Design review of the part built by this model. Coordinates are the model's own, in mm. Face numbers are marked on the shaded views. A direction names the side the tool comes from. Coordinates: 2 decimals unless noted, no trailing zeros. Write each loop counter-clockwise with the first axis right and the second up, starting at its lowest first coordinate (ties: lowest second). Pieces come first, ordered by that corner, then holes.
Q1. To check wall thickness, follow probe 1 along X at (y, z) = (5.25, -7.5); probe 2 along Y at (x, z) = (0, -1); probe 3 along X at (y, z) = (19.5, 9). State the ranges of each line that lie inside material, in increasing order.
Q2. Add section B-B, the plane z = 7.5. Give the boundary of the cut face in (x, y), plus the area to 3 significant figures.
Q3. Add section C-C, the plane y = 5.5. Give the number of separate pieces and of enclosed holes in the cut face, plus the area to 3 significant figures.
Q4. Machinability: for the marked faces 1 and 2, which of the approach directions +Z, -Z, +X, -X, +Y, -Y give a long, thin tool a straight path to every point of the face, cutting with its end or side? Answer none if there is none.
Q5. Add section A-A, the plane x = 0. Give the boundary of the cut face in (y, z).
Q6. Clearance check with flat-ended pins moving along their axes: pin 1 Ø0.6 at (x, z) = (7, 18.5) entering from -Y; pin 2 Ø2.5 at (x, y) = (-10, 19) entering from +Z; pin 3 Ø5 at (x, z) = (20, -20) entering from +Y. State where each tip first meets the part, or that it passes through.
Q7. Add section D-D, the plane z = 0. Give the boundary of the cut face in (x, y), plus the area to 3 significant figures.
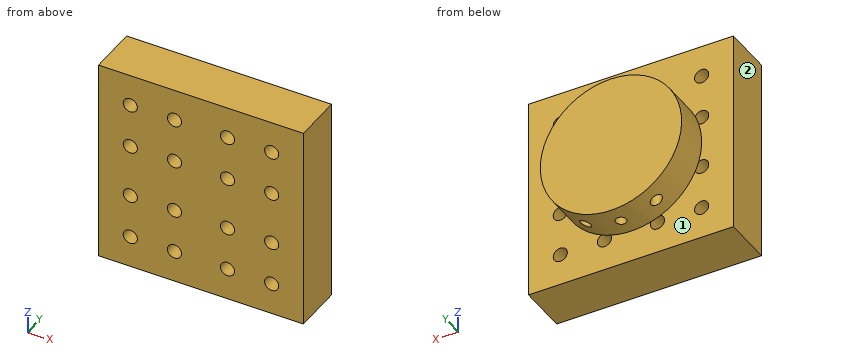
from build123d import *

# Parameters (mm, degrees)
SKETCH_4_W               = 58
SKETCH_4_H               = 58
EXTRUDE_3_DEPTH          = 14
SKETCH_6_R               = 20
EXTRUDE_4_DEPTH          = 10
CUT_EXTRUDE_1_DEPTH      = 30
CUT_EXTRUDE_1_DEPTH_BACK = 30
SKETCH_7_R               = 1.5
SKETCH_8_R               = 2
CUT_EXTRUDE_2_DEPTH      = 14


with BuildPart() as part:
    # 草图4 → 凸台-拉伸3 (new body)
    with BuildSketch(Plane(origin=(0, 0, 0), x_dir=(1, 0, 0), z_dir=(0, 1, 0))):
        Rectangle(SKETCH_4_W, SKETCH_4_H)
    extrude(amount=EXTRUDE_3_DEPTH)

    # 草图6 → 凸台-拉伸4 (add)
    with BuildSketch(Plane(origin=(0, 14, 0), x_dir=(1, 0, 0), z_dir=(0, 1, 0))):
        with Locations(Location((0, 0, 0), (0, 0, 270))):
            Circle(SKETCH_6_R)
    extrude(amount=EXTRUDE_4_DEPTH)

    # 草图7 → 切除-拉伸1 (cut, two sides: drawn at the far end of the back side and taken through both)
    with BuildSketch(Plane.XY.offset(-CUT_EXTRUDE_1_DEPTH_BACK)):
        with Locations(Location((-10, 19, 0), (0, 0, 180))):
            Circle(SKETCH_7_R)
        with Locations(Location((10, 19, 0), (0, 0, 180))):
            Circle(SKETCH_7_R)
        with Locations(Location((0, 19, 0), (0, 0, 180))):
            Circle(SKETCH_7_R)
    extrude(amount=CUT_EXTRUDE_1_DEPTH + CUT_EXTRUDE_1_DEPTH_BACK, mode=Mode.SUBTRACT)

    # 草图8 → 切除-拉伸2 (cut)
    with BuildSketch(Plane.XZ):
        with Locations(Location((-7.5, 7.5, 0), (0, 0, 270))):
            Circle(SKETCH_8_R)
        with Locations(Location((7.5, 7.5, 0), (0, 0, 270))):
            Circle(SKETCH_8_R)
        with Locations(Location((-20, 20, 0), (0, 0, 270))):
            Circle(SKETCH_8_R)
        with Locations(Location((20, 20, 0), (0, 0, 270))):
            Circle(SKETCH_8_R)
        with Locations(Location((-20, -20, 0), (0, 0, 270))):
            Circle(SKETCH_8_R)
        with Locations(Location((-7.5, -7.5, 0), (0, 0, 270))):
            Circle(SKETCH_8_R)
        with Locations(Location((7.5, -7.5, 0), (0, 0, 270))):
            Circle(SKETCH_8_R)
        with Locations(Location((20, -20, 0), (0, 0, 270))):
            Circle(SKETCH_8_R)
        with Locations(Location((-20, 7.5, 0), (0, 0, 270))):
            Circle(SKETCH_8_R)
        with Locations(Location((-20, -7.5, 0), (0, 0, 270))):
            Circle(SKETCH_8_R)
        with Locations(Location((-7.5, -20, 0), (0, 0, 270))):
            Circle(SKETCH_8_R)
        with Locations(Location((7.5, -20, 0), (0, 0, 270))):
            Circle(SKETCH_8_R)
        with Locations(Location((20, -7.5, 0), (0, 0, 270))):
            Circle(SKETCH_8_R)
        with Locations(Location((20, 7.5, 0), (0, 0, 270))):
            Circle(SKETCH_8_R)
        with Locations(Location((-7.5, 20, 0), (0, 0, 270))):
            Circle(SKETCH_8_R)
        with Locations(Location((7.5, 20, 0), (0, 0, 270))):
            Circle(SKETCH_8_R)
    extrude(amount=-CUT_EXTRUDE_2_DEPTH, mode=Mode.SUBTRACT)


solid = part.part
Here are the results:
1. probe 1: x = -29 to -22, -18 to -9.5, -5.5 to 5.5, 9.5 to 18, 22 to 29
1. probe 2: y = 0 to 17.5, 20.5 to 24
1. probe 3: x = -17.86 to -11.41, -8.59 to -1.41, 1.41 to 8.59, 11.41 to 17.86
2. outline: (-29, 0) - (-22, 0) - (-22, 14) - (-29, 14) - close; (-18.54, 14) - (-18, 14) - (-18, 0) - (-9.5, 0) - (-9.5, 14) - (-5.5, 14) - (-5.5, 0) - (5.5, 0) - (5.5, 14) - (9.5, 14) - (9.5, 0) - (18, 0) - (18, 14) - (18.54, 14) - (18.54, 24) - (-18.54, 24) - close; (22, 0) - (29, 0) - (29, 14) - (22, 14) - close; hole circle Ø3 at (-10, 19); hole circle Ø3 at (0, 19); hole circle Ø3 at (10, 19)
2. area: 938 mm2
3. separate pieces: 1
3. enclosed holes: 16
3. area: 3,160 mm2
4. face 1: +Y
4. face 2: +Z, -Z, -X, +Y, -Y
5. outline: (0, -29) - (14, -29) - (14, -20) - (17.5, -20) - (17.5, 20) - (14, 20) - (14, 29) - (0, 29) - close; (20.5, -20) - (24, -20) - (24, 20) - (20.5, 20) - close
6. pin 1: stops at y = 14
6. pin 2: passes through
6. pin 3: stops at y = 14
7. outline: (-29, 0) - (29, 0) - (29, 14) - (20, 14) - (20, 24) - (-20, 24) - (-20, 14) - (-29, 14) - close; hole circle Ø3 at (-10, 19); hole circle Ø3 at (0, 19); hole circle Ø3 at (10, 19)
7. area: 1,190 mm2
